For this review, take the finished solid that the model builds, in its own axes (mm). Give positions to 0.01 mm unless a question says otherwise; leave off trailing zeros. Write each loop counter-clockwise with the first axis right and the second up, starting at its lowest first coordinate (ties: lowest second). Pieces come first, ordered by that corner, then holes. Notation, with made-up numbers: M -35.75,-7.5 L 5.25,-7.5 A16 cw 5.25,3.5 Z; hole C 32.5,82.25 d4. An arc over 180 degrees is marked long. Use one line per item in the form item = value. Start each with the question number.
Q1. Mouldability with a two-part tool opening along Y and no side actions: class faces 1 (the flat face through (50, 1, -4)), 2 (the cylindrical face through (38.5, 9.1, -6)) as released by +Y, released by -Y, zero draft, split by the parting line, or undercut.
Q2. Consider section A-A on x = 40. Write out the cut boundary in (y, z), and give its area (3 significant figures).
Q3. For probe 1 along Y at (x, z) = (22.5, 0); probe 2 along Z at (x, y) = (26, -11); probe 3 along Y at (x, z) = (10, -6.2), list the stretches that pass through material, from the lowest coordinate up. Write a range as [from, to].
Q4. Consider section C-C on x = 7. Write out the cut boundary in (y, z).
Q5. Clearance check with flat-ended pins moving along their axes: pin 1 Ø2.5 at (x, y) = (10, 9.04) entering from -Z; pin 2 Ø1 at (x, y) = (7, 9) entering from +Z; pin 3 Ø2 at (x, z) = (35.5, -4.5) entering from +Y. State where each tip first meets the part, or that it passes through.
Q6. Consider section D-D on y = 31. Write out the cut boundary in (x, z), and give its area (3 significant figures).
Q7. Consider section B-B on z = 0. Write out the cut boundary in (x, y).
```python
from build123d import *

# Parameters (mm, degrees)
ESBO_O2_R                = 4
RESSALTO_EXTRUS_O1_DEPTH = 50
ESBO_O5_R                = 1.5
CORTE_EXTRUS_O2_DEPTH    = 40


with BuildPart() as part:
    # Esboço2 → Ressalto-extrusão1 (new body)
    with BuildSketch(Plane(origin=(0, 0, 0), x_dir=(0, 0, -1), z_dir=(1, 0, 0))):
        with BuildLine():
            Line((9, 30), (9, -30))
            ThreePointArc((9, -30), (-7.348469228, -35.196152423), (3, -21.514718626))
            Line((3, -21.514718626), (3, 21.514718626))
            ThreePointArc((3, 21.514718626), (-7.348469228, 35.196152423), (9, 30))
        make_face()
        with Locations((0, 30)):
            Circle(ESBO_O2_R, mode=Mode.SUBTRACT)
        with Locations((0, -30)):
            Circle(ESBO_O2_R, mode=Mode.SUBTRACT)
    extrude(amount=RESSALTO_EXTRUS_O1_DEPTH)

    # Esboço5 → Corte-extrusão2 (cut)
    with BuildSketch(Plane.XY.offset(-3)):
        with Locations((10, 9.044428523)):
            Circle(ESBO_O5_R)
        with Locations((40, 9.044428523)):
            Circle(ESBO_O5_R)
        with Locations((40, -9.044428523)):
            Circle(ESBO_O5_R)
        with Locations((10, -9.044428523)):
            Circle(ESBO_O5_R)
    extrude(amount=-CORTE_EXTRUS_O2_DEPTH, mode=Mode.SUBTRACT)


solid = part.part
```
Working result:
q1.face_1 = zero draft
q1.face_2 = undercut
q2.outline = M -30,-9 L -10.54,-9 L -10.54,-3 L -21.51,-3 A9 ccw long Z; M -7.54,-9 L 7.54,-9 L 7.54,-3 L -7.54,-3 Z; M 10.54,-9 L 30,-9 A9 ccw long 21.51,-3 L 10.54,-3 Z; hole C -30,0 d8; hole C 30,0 d8
q2.area = 658 mm²
q3.probe_1 = [-39, -34], [-26, -21], [21, 26], [34, 39]
q3.probe_2 = [-9, -3]
q3.probe_3 = [-36.52, -10.54], [-7.54, 7.54], [10.54, 36.52]
q4.outline = M -30,-9 L 30,-9 A9 ccw long 21.51,-3 L -21.51,-3 A9 ccw long Z; hole C -30,0 d8; hole C 30,0 d8
q5.pin_1 = through
q5.pin_2 = -3
q5.pin_3 = 38.29
q6.outline = M 0,-8.94 L 50,-8.94 L 50,-3.87 L 0,-3.87 Z; M 0,3.87 L 50,3.87 L 50,8.94 L 0,8.94 Z
q6.area = 507 mm²
q7.outline = M 0,-39 L 50,-39 L 50,-34 L 0,-34 Z; M 0,-26 L 50,-26 L 50,-21 L 0,-21 Z; M 0,21 L 50,21 L 50,26 L 0,26 Z; M 0,34 L 50,34 L 50,39 L 0,39 Z
